Geometry: final body of the model. Coordinates: model frame, mm. A direction names the side the tool comes from. Give positions to 0.01 mm unless a question says otherwise; leave off trailing zeros. Write each loop counter-clockwise with the first axis right and the second up, starting at its lowest first coordinate (ties: lowest second). Pieces come first, ordered by that corner, then holes. Notation, with made-up numbers: (47, 54.25) -> (94, 54.25) arc R22 ccw to (94, 88.25) -> close; hole circle Ø2 at (34.5, 84.5). An arc over 180 degrees is marked (long way). Answer in a Markdown table with one row per item. Add a question column.
Item 1: Material intervals for probe 1 along Z at (x, y) = (-14.5, 0.6); probe 2 along Z at (x, y) = (-0.7, 0.5); probe 3 along X at (y, z) = (0.3, 2.54), sorted ascending. Write a range as from..to.
Item 2: Section query D-D on x = 10. Output: boundary loops of the cut face in (y, z), plus the area to 3 significant figures.
Item 3: Section query B-B on x = -0.7. Output: boundary loops of the cut face in (y, z).
Item 4: First-contact query: P1, Ø4, axis at x = 6, y = 8, coming from the -Z side; P2, Ø0.6, axis at x = 10, z = -0.5, coming from the +Y side. Flat tips, straight axial feed; report the tip coordinate or a pass-through.
Item 5: Draft query along Z for faces 1 (the flat face through (-0.2, 0.5, 6.5)), 2 (the cylindrical face through (-14.023, 0.507, 2.39)), 3 (the flat face through (-16, 0.5, 0.1)). Return one class per face: +Z half, -Z half, draft (parallel to the pull), parting line (faces both ways), or undercut.
Item 6: Access query for faces 4 (the flat face through (-0.2, 0.5, -6.5)), 5 (the cylindrical face through (9.2, 9, 0.6)). Directions: +Z, -Z, +X, -X, +Y, -Y. A direction counts if a zero-diameter tool reaches every point of the face in a straight line with its end or side. Return the directions, or none.
Item 7: Section query C-C on z = 2.54. Output: boundary loops of the cut face in (x, y), plus the area to 3 significant figures.
Item 8: Section query A-A on x = -14.5. Output: boundary loops of the cut face in (y, z).
```python
from build123d import *

# Parameters (mm, degrees)
SKETCH_1_W          = 32
SKETCH_1_H          = 13
EXTRUDE_1_DEPTH     = 1
SKETCH_2_R          = 1.75
CUT_EXTRUDE_1_DEPTH = 2
EXTRUDE_START       = -1
SKETCH_4_R          = 6
EXTRUDE_2_DEPTH     = 10
SKETCH_5_R          = 0.5
CUT_EXTRUDE_2_DEPTH = 2
SKETCH_6_R          = 1
CUT_EXTRUDE_3_DEPTH = 2


with BuildPart() as part:
    # 草图1 → 凸台-拉伸1 (new body)
    with BuildSketch(Plane(origin=(0, 0, 0), x_dir=(1, 0, 0), z_dir=(0, 1, 0))):
        Rectangle(SKETCH_1_W, SKETCH_1_H)
    extrude(amount=EXTRUDE_1_DEPTH)

    # 草图2 → 切除-拉伸1 (cut, through all)
    with BuildSketch(Plane(origin=(0, 1, 0), x_dir=(1, 0, 0), z_dir=(0, 1, 0))):
        with Locations((-0.7, 0)):
            Circle(SKETCH_2_R)
    extrude(amount=-CUT_EXTRUDE_1_DEPTH, mode=Mode.SUBTRACT)

    # 草图4 → 凸台-拉伸2 (add)
    with BuildSketch(Plane(origin=(0, 1, 0), x_dir=(1, 0, 0), z_dir=(0, 1, 0)).offset(EXTRUDE_START)):
        with Locations((10, 0)):
            Circle(SKETCH_4_R)
    extrude(amount=EXTRUDE_2_DEPTH)

    # 草图5 → 切除-拉伸2 (cut, through all)
    with BuildSketch(Plane(origin=(0, 1, 0), x_dir=(1, 0, 0), z_dir=(0, 1, 0))):
        with Locations((-14.5, 2.54)):
            Circle(SKETCH_5_R)
        with Locations((-14.5, 0)):
            Circle(SKETCH_5_R)
        with Locations((-14.5, -2.54)):
            Circle(SKETCH_5_R)
    extrude(amount=-CUT_EXTRUDE_2_DEPTH, mode=Mode.SUBTRACT)

    # 草图6 → 切除-拉伸3 (cut)
    with BuildSketch(Plane(origin=(0, 10, 0), x_dir=(1, 0, 0), z_dir=(0, 1, 0))):
        with Locations((10, 0)):
            Circle(SKETCH_6_R)
    extrude(amount=-CUT_EXTRUDE_3_DEPTH, mode=Mode.SUBTRACT)


solid = part.part
```
Findings below:
| question | item | result |
|---|---|---|
| 1 | probe 1 | z = -6.5..-3.04, -2.04..-0.5, 0.5..2.04, 3.04..6.5 |
| 1 | probe 2 | z = -6.5..-1.75, 1.75..6.5 |
| 1 | probe 3 | x = -16..-15, -14..16 |
| 2 | outline | (0, -6.5) -> (1, -6.5) -> (1, -6) -> (10, -6) -> (10, -1) -> (8, -1) -> (8, 1) -> (10, 1) -> (10, 6) -> (1, 6) -> (1, 6.5) -> (0, 6.5) -> close |
| 2 | area | 117 mm^2 |
| 3 | outline | (0, -6.5) -> (1, -6.5) -> (1, -1.75) -> (0, -1.75) -> close; (0, 1.75) -> (1, 1.75) -> (1, 6.5) -> (0, 6.5) -> close |
| 4 | P1 | stops at z = -5.66 |
| 4 | P2 | stops at y = 8 |
| 5 | face 1 | +Z half |
| 5 | face 2 | undercut |
| 5 | face 3 | draft |
| 6 | face 4 | -Z, +X, -X, +Y, -Y |
| 6 | face 5 | +Y |
| 7 | outline | (-16, 0) -> (-15, 0) -> (-15, 1) -> (-16, 1) -> close; (-14, 0) -> (16, 0) -> (16, 1) -> (15.44, 1) -> (15.44, 10) -> (4.56, 10) -> (4.56, 1) -> (-14, 1) -> close |
| 7 | area | 129 mm^2 |
| 8 | outline | (0, -6.5) -> (1, -6.5) -> (1, -3.04) -> (0, -3.04) -> close; (0, -2.04) -> (1, -2.04) -> (1, -0.5) -> (0, -0.5) -> close; (0, 0.5) -> (1, 0.5) -> (1, 2.04) -> (0, 2.04) -> close; (0, 3.04) -> (1, 3.04) -> (1, 6.5) -> (0, 6.5) -> close |
